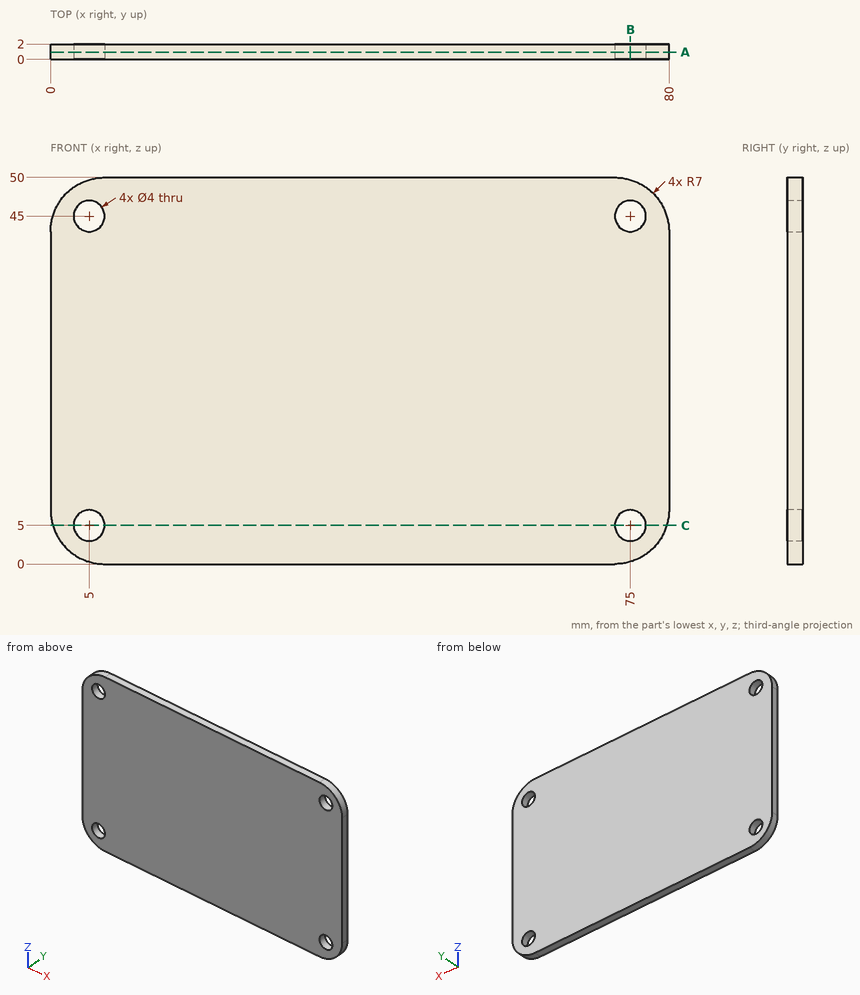
Check sheet for the drawn part. Datum: minimum x, y, z corner. Units: mm. Round coordinates to 2 decimals unless told otherwise and drop trailing zeros. Order: outer loops, then holes, each group sorted by start corner. A loop starts at its lowest first (then second) coordinate and runs counter-clockwise, first axis right, second up. Notation, with made-up numbers: (13, -16) -> (37, -16) arc R15 ccw to (37, -1) -> close; hole circle Ø5 at (34, 74). An arc over 180 degrees is marked (long way). Put each result on its own line as item: value. Start each with the question number.
(1) Material ranges on line 1 along X through (y, z) = (0.55, 45); line 2 along Z through (x, y) = (6, 0.1); line 3 along Z through (x, y) = (75, 0.9), recorded low to high.
(2) Section check C-C (z = 5). Enter the section's corners in (x, y), then the cut area to 3 significant figures.
(3) Depth check by flat-ended pin: pin 1 Ø3 at (x, z) = (75, 45) entering from -Y. Enter the tip coordinate at first touch or a pass-through.
(4) Section check A-A (y = 0.95). Enter the section's corners in (x, z).
(5) Section check B-B (x = 75). Enter the section's corners in (y, z), then the cut area to 3 significant figures.
Completed:
1. line 1: x = 0.29 to 3, 7 to 73, 77 to 79.71
1. line 2: z = 0.07 to 3.27, 6.73 to 43.27, 46.73 to 49.93
1. line 3: z = 0.29 to 3, 7 to 43, 47 to 49.71
2. outline: (0.29, 0) -> (3, 0) -> (3, 2) -> (0.29, 2) -> close; (7, 0) -> (73, 0) -> (73, 2) -> (7, 2) -> close; (77, 0) -> (79.71, 0) -> (79.71, 2) -> (77, 2) -> close
2. area: 143 mm2
3. pin 1: passes through
4. outline: (0, 7) arc R7 ccw to (7, 0) -> (73, 0) arc R7 ccw to (80, 7) -> (80, 43) arc R7 ccw to (73, 50) -> (7, 50) arc R7 ccw to (0, 43) -> close; hole circle Ø4 at (5, 5); hole circle Ø4 at (5, 45); hole circle Ø4 at (75, 5); hole circle Ø4 at (75, 45)
5. outline: (0, 0.29) -> (2, 0.29) -> (2, 3) -> (0, 3) -> close; (0, 7) -> (2, 7) -> (2, 43) -> (0, 43) -> close; (0, 47) -> (2, 47) -> (2, 49.71) -> (0, 49.71) -> close
5. area: 82.8 mm2
